For this review, take the finished solid that the model builds, in its own axes (mm). A direction names the side the tool comes from. Give positions to 0.01 mm unless a question says otherwise; leave off trailing zeros. Loops run counter-clockwise (first coordinate to the right, second up) from the corner with the lowest first, then second, coordinate; pieces in that order, holes last.
```python
from build123d import *

# Parameters (mm, degrees)
SKETCH_1_R      = 2.5
SKETCH_1_W      = 14.25
SKETCH_1_H      = 1.5
EXTRUDE_2_DEPTH = 5.5


with BuildPart() as part:
    # 草圖1 → 填料-伸長2 (new body)
    with BuildSketch(Plane.XY):
        Polygon((-70.969139755, -35.192052365), (-85.219139755, -35.192052365), (-85.219139755, -35.633297351), (-85.219139755, -36.892052365), (-73.216342126, -36.014419398), (-73.216342126, -54.369685333), (-85.219139755, -53.692052365), (-85.219139755, -54.75080738), (-85.219139755, -55.192052365), (-85.219139755, -56.692052365), (-70.969139755, -56.692052365), (-70.969139755, -55.192052365), (-70.969139755, -48.592052365), (-66.164139755, -48.592052365), (-29.469139755, -48.592052365), (-29.469139755, -55.192052365), (-29.469139755, -56.692052365), (-15.219139755, -56.692052365), (-15.219139755, -55.192052365), (-15.219139755, -54.75080738), (-15.219139755, -53.692052365), (-27.221937385, -54.369685333), (-27.221937385, -36.014419398), (-15.219139755, -36.892052365), (-15.219139755, -35.633297351), (-15.219139755, -35.192052365), (-15.219139755, -33.692052365), (-29.469139755, -33.692052365), (-29.469139755, -35.192052365), (-29.469139755, -41.792052365), (-66.164139755, -41.792052365), (-70.969139755, -41.792052365), align=None)
        with Locations((-66.164139755, -45.192052365)):
            Circle(SKETCH_1_R, mode=Mode.SUBTRACT)
        with Locations((-58.194139755, -45.192052365)):
            Circle(SKETCH_1_R, mode=Mode.SUBTRACT)
        with Locations((-50.224139755, -45.192052365)):
            Circle(SKETCH_1_R, mode=Mode.SUBTRACT)
        with Locations((-42.254139755, -45.192052365)):
            Circle(SKETCH_1_R, mode=Mode.SUBTRACT)
        with Locations((-34.284139755, -45.192052365)):
            Circle(SKETCH_1_R, mode=Mode.SUBTRACT)
        with Locations((-78.094139755, -34.442052365)):
            Rectangle(SKETCH_1_W, SKETCH_1_H)
    extrude(amount=EXTRUDE_2_DEPTH)


solid = part.part
```
Item 1: Take a section at C-C on z = 2.9. Give the boundary of the cut face in (x, y).
Answer:
outline: (-85.22, -56.69) - (-70.97, -56.69) - (-70.97, -48.59) - (-29.47, -48.59) - (-29.47, -56.69) - (-15.22, -56.69) - (-15.22, -53.69) - (-27.22, -54.37) - (-27.22, -36.01) - (-15.22, -36.89) - (-15.22, -33.69) - (-29.47, -33.69) - (-29.47, -41.79) - (-70.97, -41.79) - (-70.97, -33.69) - (-85.22, -33.69) - (-85.22, -36.89) - (-73.22, -36.01) - (-73.22, -54.37) - (-85.22, -53.69) - close; hole circle Ø5 at (-66.16, -45.19); hole circle Ø5 at (-58.19, -45.19); hole circle Ø5 at (-50.22, -45.19); hole circle Ø5 at (-42.25, -45.19); hole circle Ø5 at (-34.28, -45.19)
Item 2: Take a section at A-A on y = -37.75. Give the boundary of the cut face in (x, z).
Answer:
outline: (-73.22, 0) - (-70.97, 0) - (-70.97, 5.5) - (-73.22, 5.5) - close; (-29.47, 0) - (-27.22, 0) - (-27.22, 5.5) - (-29.47, 5.5) - close
Item 3: Tool access review of faces 4 (the flat face through (-21.305, -36.447, 2.712)), 5 (the flat face through (-85.219, -35, 3)), 6 (the flat face through (-29.469, -38, 3)), 7 (the flat face through (-70.969, -53, 3)), 8 (the flat face through (-78, -56.692, 3)): name each direction out of +Z, -Z, +X, -X, +Y, -Y from which nothing blocks a thin tool from reaching the whole face with its end or side.
Answer:
face 4: +Z, -Z
face 5: +Z, -Z, -X, +Y, -Y
face 6: +Z, -Z, +Y
face 7: +Z, -Z, -Y
face 8: +Z, -Z, +X, -X, -Y
Item 4: Take a section at D-D on y = -47. Give the boundary of the cut face in (x, z).
Answer:
outline: (-73.22, 0) - (-67.89, 0) - (-67.89, 5.5) - (-73.22, 5.5) - close; (-64.44, 0) - (-59.92, 0) - (-59.92, 5.5) - (-64.44, 5.5) - close; (-56.47, 0) - (-51.95, 0) - (-51.95, 5.5) - (-56.47, 5.5) - close; (-48.5, 0) - (-43.98, 0) - (-43.98, 5.5) - (-48.5, 5.5) - close; (-40.53, 0) - (-36.01, 0) - (-36.01, 5.5) - (-40.53, 5.5) - close; (-32.56, 0) - (-27.22, 0) - (-27.22, 5.5) - (-32.56, 5.5) - close
Item 5: The part is to be moulded in two halves that separate along Y. For faces 1 (the flat face through (-22, -33.692, 3)), 2 (the cylindrical face through (-36.78, -45.08, 2.71)), 3 (the flat face through (-22, -56.692, 3)), say which applies: released by +Y, released by -Y, zero draft, split by the parting line, or undercut.
Answer:
face 1: released by +Y
face 2: undercut
face 3: released by -Y
Item 6: Clearance check with flat-ended pins moving along their axes: pin 1 Ø1.5 at (x, z) = (-59.5, 3) entering from -Y; pin 2 Ø1 at (y, z) = (-41, 1.5) entering from +X; pin 3 Ø3 at (y, z) = (-39, 3) entering from -X; pin 4 Ø4.5 at (x, y) = (-34.28, -45.19) entering from -Z. State where each tip first meets the part, or that it passes through.
Answer:
pin 1: stops at y = -48.59
pin 2: stops at x = -27.22
pin 3: stops at x = -73.22
pin 4: passes through
Item 7: For L1, parallel to X at y = -39.5, z = 5.15; L2, parallel to X at y = -45.25, z = 1.7; L3, parallel to X at y = -46.5, z = 5.2, list the stretches that pass through material, from the lowest coordinate up.
Answer:
L1: x = -73.22 to -70.97, -29.47 to -27.22
L2: x = -73.22 to -68.66, -63.66 to -60.69, -55.69 to -52.72, -47.72 to -44.75, -39.75 to -36.78, -31.78 to -27.22
L3: x = -73.22 to -68.29, -64.03 to -60.32, -56.06 to -52.35, -48.09 to -44.38, -40.12 to -36.41, -32.15 to -27.22
Item 8: Take a section at B-B on x = -56.5. Give the boundary of the cut face in (y, z).
Answer:
outline: (-48.59, 0) - (-47.03, 0) - (-47.03, 5.5) - (-48.59, 5.5) - close; (-43.35, 0) - (-41.79, 0) - (-41.79, 5.5) - (-43.35, 5.5) - close
